The listing builds one solid part. Answer for the finished solid, in the listing's coordinates (mm). A direction names the side the tool comes from. Coordinates: 2 decimals unless noted, no trailing zeros. Write each loop counter-clockwise with the first axis right and the second up, starting at its lowest first coordinate (ties: lowest second). Pieces come first, ordered by that corner, then holes.
from build123d import *

# Parameters (mm, degrees)
BOSS_EXTRUDE1_DEPTH = 50.8
CUT_EXTRUDE1_REACH  = 75.66
SKETCH12_R          = 3.175


with BuildPart() as part:
    # Sketch11 → Boss-Extrude1 (new body)
    with BuildSketch(Plane.XY):
        Polygon((0, 0), (38.1, 0), (38.1, 71.12), (96.52, 71.12), (96.52, 0), (134.62, 0), (134.62, 2.54), (99.06, 2.54), (99.06, 73.66), (35.56, 73.66), (35.56, 2.54), (0, 2.54), align=None)
    extrude(amount=-BOSS_EXTRUDE1_DEPTH)

    # Sketch12 → Cut-Extrude1 (cut, up to next)
    with BuildSketch(Plane(origin=(0, 73.66, 0), x_dir=(1, 0, 0), z_dir=(0, 1, 0)), mode=Mode.PRIVATE) as cut_extrude1_sk1:
        with Locations((43.18, 10.16)):
            Circle(SKETCH12_R)
    cut_extrude1_tool1 = extrude(cut_extrude1_sk1.sketch, amount=-CUT_EXTRUDE1_REACH, mode=Mode.PRIVATE) & part.part
    add(cut_extrude1_tool1.solids().sort_by_distance((43.18, 73.66, -10.16))[0], mode=Mode.SUBTRACT)
    # Sketch12 → Cut-Extrude1 (cut, up to next)
    with BuildSketch(Plane(origin=(0, 73.66, 0), x_dir=(1, 0, 0), z_dir=(0, 1, 0)), mode=Mode.PRIVATE) as cut_extrude1_sk2:
        with Locations((91.44, 10.16)):
            Circle(SKETCH12_R)
    cut_extrude1_tool2 = extrude(cut_extrude1_sk2.sketch, amount=-CUT_EXTRUDE1_REACH, mode=Mode.PRIVATE) & part.part
    add(cut_extrude1_tool2.solids().sort_by_distance((91.44, 73.66, -10.16))[0], mode=Mode.SUBTRACT)
    # Sketch12 → Cut-Extrude1 (cut, up to next)
    with BuildSketch(Plane(origin=(0, 73.66, 0), x_dir=(1, 0, 0), z_dir=(0, 1, 0)), mode=Mode.PRIVATE) as cut_extrude1_sk3:
        with Locations((91.44, 40.64)):
            Circle(SKETCH12_R)
    cut_extrude1_tool3 = extrude(cut_extrude1_sk3.sketch, amount=-CUT_EXTRUDE1_REACH, mode=Mode.PRIVATE) & part.part
    add(cut_extrude1_tool3.solids().sort_by_distance((91.44, 73.66, -40.64))[0], mode=Mode.SUBTRACT)
    # Sketch12 → Cut-Extrude1 (cut, up to next)
    with BuildSketch(Plane(origin=(0, 73.66, 0), x_dir=(1, 0, 0), z_dir=(0, 1, 0)), mode=Mode.PRIVATE) as cut_extrude1_sk4:
        with Locations((43.18, 40.64)):
            Circle(SKETCH12_R)
    cut_extrude1_tool4 = extrude(cut_extrude1_sk4.sketch, amount=-CUT_EXTRUDE1_REACH, mode=Mode.PRIVATE) & part.part
    add(cut_extrude1_tool4.solids().sort_by_distance((43.18, 73.66, -40.64))[0], mode=Mode.SUBTRACT)


solid = part.part
Q1. The part is cut by section B-B, the plane z = -10.16. Write down the section's boundary in (x, y) (3 decimals).
Answers below:
outline: (0, 0) - (38.1, 0) - (38.1, 71.12) - (40.005, 71.12) - (40.005, 73.66) - (35.56, 73.66) - (35.56, 2.54) - (0, 2.54) - close; (46.355, 71.12) - (88.265, 71.12) - (88.265, 73.66) - (46.355, 73.66) - close; (94.615, 71.12) - (96.52, 71.12) - (96.52, 0) - (134.62, 0) - (134.62, 2.54) - (99.06, 2.54) - (99.06, 73.66) - (94.615, 73.66) - close
Q2. Given pin 1 (10.5 mm diameter, centred on x = 109.5, z = -13, fed in from +Y); pin 2 (10 mm diameter, centred on x = 105, y = 23.5, fed in from -Z); pin 3 (1.5 mm diameter, centred on x = 96.5, z = -14, fed in from -Y); pin 4 (12 mm diameter, centred on x = 54.5, z = -18.5, fed in from -Y), each flat-ended and moving along its own axis, determine where each tip first touches the part or whether it passes through.
Answers below:
pin 1: stops at y = 2.54
pin 2: passes through
pin 3: stops at y = 0
pin 4: stops at y = 71.12
Q3. The part is cut by section A-A, the plane x = 91.44. Write down the section's boundary in (y, z) (3 decimals).
Answers below:
outline: (71.12, -50.8) - (73.66, -50.8) - (73.66, -43.815) - (71.12, -43.815) - close; (71.12, -37.465) - (73.66, -37.465) - (73.66, -13.335) - (71.12, -13.335) - close; (71.12, -6.985) - (73.66, -6.985) - (73.66, 0) - (71.12, 0) - close
Q4. Find the intervals of material crossed by probe 1 along X at (y, z) = (72.5, -10.16) (3 decimals); probe 2 along Z at (x, y) = (43, 72); probe 3 along X at (y, z) = (23, -25), in increasing order.
Answers below:
probe 1: x = 35.56 to 40.005, 46.355 to 88.265, 94.615 to 99.06
probe 2: z = -50.8 to -43.81, -37.47 to -13.33, -6.99 to 0
probe 3: x = 35.56 to 38.1, 96.52 to 99.06
Q5. Which of the six approach directions +Z, -Z, +X, -X, +Y, -Y give full straight-line access (tool end or side, diameter ignored) to faces 4 (the face through (40.01, 72.41, -10.3)), 5 (the face through (35.56, 39, -25)), 6 (the face through (99.06, 38, -25)), 7 (the face through (38.1, 35, -25))?
Answers below:
face 4: +Y, -Y
face 5: +Z, -Z, -X, +Y
face 6: +Z, -Z, +X, +Y
face 7: +Z, -Z, -Y
Q6. The part is cut by section C-C, the plane y = 66.5. Write down the section's boundary in (x, z), then the cut area to 3 significant figures.
Answers below:
outline: (35.56, -50.8) - (38.1, -50.8) - (38.1, 0) - (35.56, 0) - close; (96.52, -50.8) - (99.06, -50.8) - (99.06, 0) - (96.52, 0) - close
area: 258 mm2
Q7. Determine the mould class of faces 1 (the face through (97, 37, 0)), 2 (the face through (88.92, 72.41, -38.71)), 3 (the face through (115, 0, -25)) for opening direction Z: released by +Z, released by -Z, zero draft, split by the parting line, or undercut.
Answers below:
face 1: released by +Z
face 2: undercut
face 3: zero draft
Q8. The part is cut by section D-D, the plane z = -4. Write down the section's boundary in (x, y), then the cut area to 3 significant figures.
Answers below:
outline: (0, 0) - (38.1, 0) - (38.1, 71.12) - (96.52, 71.12) - (96.52, 0) - (134.62, 0) - (134.62, 2.54) - (99.06, 2.54) - (99.06, 73.66) - (35.56, 73.66) - (35.56, 2.54) - (0, 2.54) - close
area: 703 mm2
